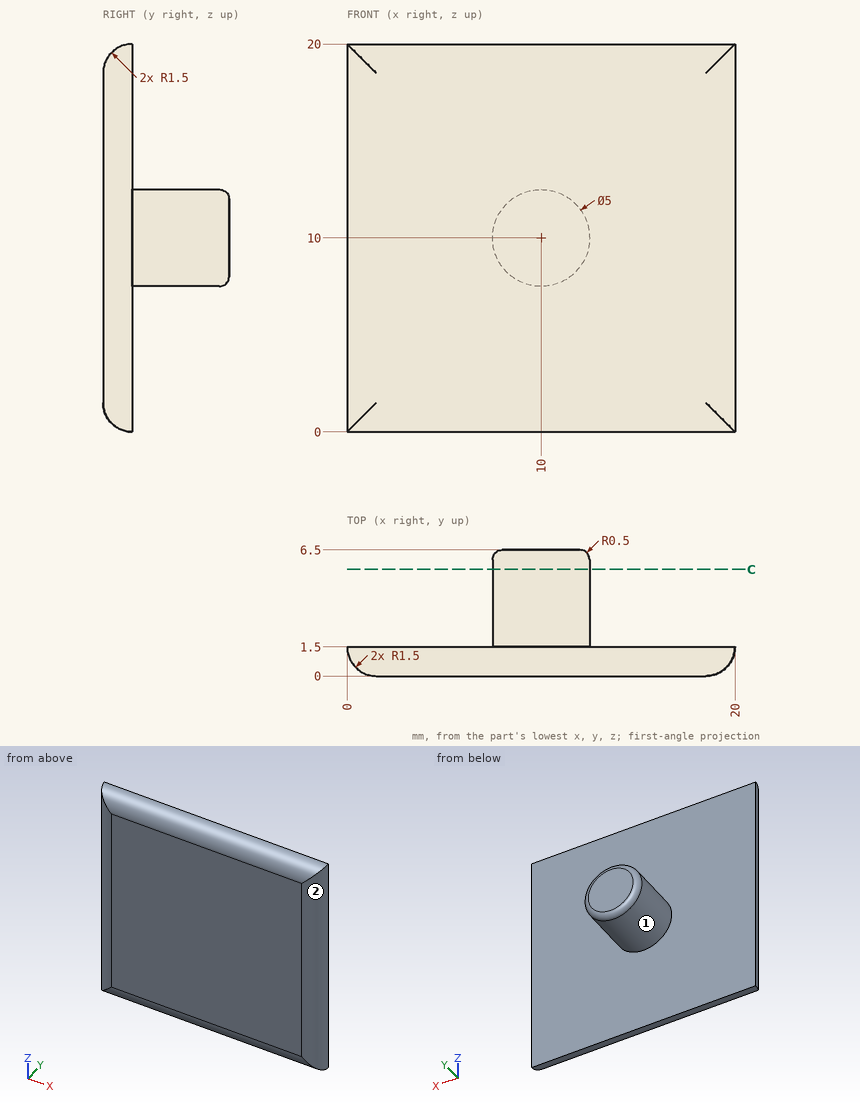
Geometry: see drawing. Coordinates: mm, zero at the bounding-box minimum. A direction names the side the tool comes from. Round coordinates to 2 decimals unless told otherwise and drop trailing zeros. Loops run counter-clockwise (first coordinate to the right, second up) from the corner with the lowest first, then second, coordinate; pieces in that order, holes last. Notation, with made-up numbers: (-36.5, 53) - (-21.5, 53) arc R25 cw to (-21.5, 70) - close; hole circle Ø5 at (-21.5, 79). An arc over 180 degrees is marked (long way). One line per item, written item: value. Start each with the question number.
(1) Contact query for flat-ended pins moving along their axis: P1, Ø3, axis at y = 4, z = 7.5, coming from the -X side; P2, Ø1, axis at x = 11.5, y = 4.5, coming from the +Z side; P3, Ø4, axis at x = 5, z = 6.5, coming from the +Y side. Output: stop coordinate, or through.
(2) Ray query, line 1 (Y direction, x = 8.5, z = 12.5); line 2 (X direction, y = 4, z = 11.5); line 3 (X direction, y = 1.25, z = 7.25). Return the intervals inside material, ascending. Write a range as [from, to].
(3) Section C-C, the plane y = 5.5. Return loops of the section in (x, z), plus the area to 3 significant figures.
(4) Access query for the marked faces 1 and 2. Directions: +Z, -Z, +X, -X, +Y, -Y. A direction counts if a zero-diameter tool reaches every point of the face in a straight line with its end or side. Return the directions, or none.
Results below:
1. P1: x = 7.71
1. P2: z = 12.29
1. P3: y = 1.5
2. line 1: [0, 1.5]
2. line 2: [8, 12]
2. line 3: [0.02, 19.98]
3. outline: circle Ø5 at (10, 10)
3. area: 19.6 mm^2
4. face 1: +Y
4. face 2: +Z, -Z, +X, -Y
